The listing builds one solid part. Answer for the finished solid, in the listing's coordinates (mm). A direction names the side the tool comes from. Round coordinates to 2 decimals unless told otherwise and drop trailing zeros. Order: outer loops, then holes, each group sorted by start corner. A loop starts at its lowest first (then second) coordinate and runs counter-clockwise, first axis right, second up. Notation, with made-up numbers: (45.5, 39.5) - (83.5, 39.5) arc R26 cw to (83.5, 56.5) - close; hole circle Ø6 at (15.25, 23.5). An arc over 180 degrees is marked (long way). One line per item, written item: value. Start each with the question number.
1. A tool of negligible diameter and unlimited length cuts with its end or side. For faces 1 (the flat face through (6.35, -9, 1)), 2 (the flat face through (-6.172, -3.219, -5.474)), from which of +Z, -Z, +X, -X, +Y, -Y can it reach the whole face along a straight path? Write none if from no direction.
2. Section A-A, the plane z = 0 is taken. Give the vertices of the cut face in (x, y), then the cut area to 3 significant figures.
3. Section D-D, the plane z = -10 is taken. Give the vertices of the cut face in (x, y), then the cut area to 3 significant figures.
4. Section C-C, the plane x = -12.7 is taken. Give the vertices of the cut face in (y, z), then the cut area to 3 significant figures.
5. For a pull along Z with two mould halves and no side action, classify faces 3 (the flat face through (0, 11, 30)), 4 (the flat face through (-6.172, 3.131, -5.525)), 5 (the cylindrical face through (-9.392, -30.995, 6.883)) as released by +Z, released by -Z, zero draft, split by the parting line, or undercut.
6. Section B-B, the plane y = 25.5 is taken. Give the vertices of the cut face in (x, z).
7. Straight lines are drawn through the part: line 1 (X direction, y = -26, z = 0); line 2 (X direction, y = 38, z = 0); line 3 (Z direction, x = -10, y = -14). For each, find the intervals that lie inside material, in ascending order.
8. Flat-ended cylindrical pins translate along their axes: P1, Ø10, axis at x = -6.5, y = -26, coming from the -Z side; P2, Ø2, axis at x = -3.5, z = 0, coming from the +Y side; P3, Ø8, axis at x = 1.5, y = -8, coming from the +Z side. Find the tip coordinate at first contact, or state that the pin passes through.
from build123d import *

# Parameters (mm, degrees)
SKETCH1_R               = 44.45
BOSS_EXTRUDE1_DEPTH     = 6.35
SKETCH2_R               = 31.75
BOSS_EXTRUDE2_DEPTH     = 19.05
CUT_EXTRUDE1_DEPTH      = 66.684910748
CUT_EXTRUDE1_DEPTH_BACK = 66.684910748
SKETCH3_R               = 3.139622981


with BuildPart() as part:
    # Sketch1 → Boss-Extrude1 (new body)
    with BuildSketch(Plane(origin=(0, 0, 0), x_dir=(0, 0, -1), z_dir=(1, 0, 0))):
        Circle(SKETCH1_R)
        Polygon((3.666174209, -6.35), (7.332348419, 0), (3.666174209, 6.35), (-3.666174209, 6.35), (-7.332348419, 0), (-3.666174209, -6.35), align=None, mode=Mode.SUBTRACT)
    extrude(amount=BOSS_EXTRUDE1_DEPTH)

    # Sketch2 → Boss-Extrude2 (add)
    with BuildSketch(Plane(origin=(0, 0, 0), x_dir=(0, 0, -1), z_dir=(1, 0, 0))):
        Circle(SKETCH2_R)
        Polygon((-7.332348419, 0), (-3.666174209, -6.35), (3.666174209, -6.35), (7.332348419, 0), (3.666174209, 6.35), (-3.666174209, 6.35), align=None, mode=Mode.SUBTRACT)
    extrude(amount=-BOSS_EXTRUDE2_DEPTH)

    # Sketch3 → Cut-Extrude1 (cut, two sides: drawn at the far end of the back side and taken through both)
    with BuildSketch(Plane(origin=(0, 0, 0), x_dir=(1, 0, 0), z_dir=(0, 1, 0)).offset(-CUT_EXTRUDE1_DEPTH_BACK)):
        with Locations(Location((-12.7, 0, 0), (0, 0, 270))):
            Circle(SKETCH3_R)
    extrude(amount=CUT_EXTRUDE1_DEPTH + CUT_EXTRUDE1_DEPTH_BACK, mode=Mode.SUBTRACT)


solid = part.part
Answer list:
1. face 1: +Z, -Z, +X, +Y, -Y
1. face 2: +X, -X
2. outline: (-19.05, -31.75) - (-15.84, -31.75) - (-15.84, -6.35) - (-19.05, -6.35) - close; (-19.05, 6.35) - (-15.84, 6.35) - (-15.84, 31.75) - (-19.05, 31.75) - close; (-9.56, -31.75) - (0, -31.75) - (0, -44.45) - (6.35, -44.45) - (6.35, -6.35) - (-9.56, -6.35) - close; (-9.56, 6.35) - (6.35, 6.35) - (6.35, 44.45) - (0, 44.45) - (0, 31.75) - (-9.56, 31.75) - close
2. area: 1,130 mm²
3. outline: (-19.05, -30.13) - (0, -30.13) - (0, -43.31) - (6.35, -43.31) - (6.35, 43.31) - (0, 43.31) - (0, 30.13) - (-19.05, 30.13) - close
3. area: 1,700 mm²
4. outline: (-31.59, -3.14) arc R31.75 ccw to (31.59, -3.14) - (6.35, -3.14) - (6.35, -3.67) - (0, -7.33) - (-6.35, -3.67) - (-6.35, -3.14) - close; (-31.59, 3.14) - (-6.35, 3.14) - (-6.35, 3.67) - (0, 7.33) - (6.35, 3.67) - (6.35, 3.14) - (31.59, 3.14) arc R31.75 ccw to start
4. area: 2,710 mm²
5. face 3: zero draft
5. face 4: undercut
5. face 5: split by the parting line
6. outline: (-19.05, -18.92) - (0, -18.92) - (0, -36.41) - (6.35, -36.41) - (6.35, 36.41) - (0, 36.41) - (0, 18.92) - (-19.05, 18.92) - close; hole circle Ø6.28 at (-12.7, 0)
7. line 1: x = -19.05 to -15.84, -9.56 to 6.35
7. line 2: x = 0 to 6.35
7. line 3: z = -28.5 to -1.6, 1.6 to 28.5
8. P1: stops at z = -23.81
8. P2: stops at y = 31.75
8. P3: stops at z = 44.27
